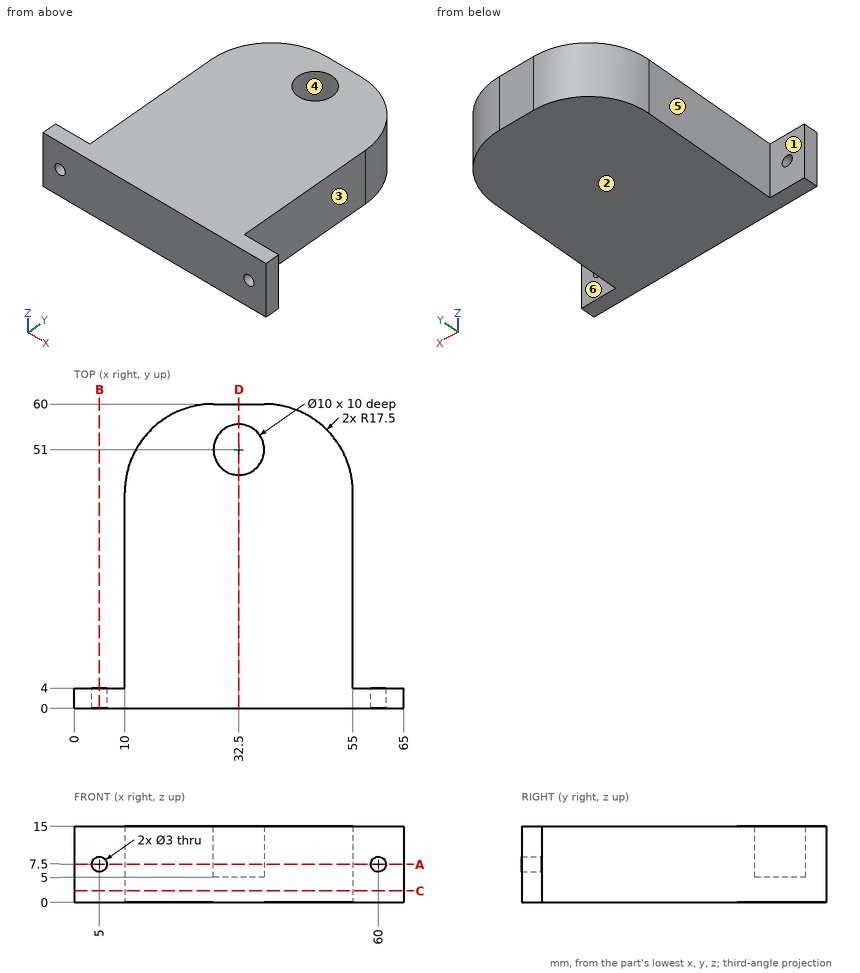
Here's the drawing with two shaded views (mm, measured from the low corner). I have some questions. A direction names the side the tool comes from. Give positions to 0.01 mm unless a question says otherwise; leave off trailing zeros. Order: outer loops, then holes, each group sorted by start corner. A loop starts at its lowest first (then second) coordinate and runs counter-clockwise, first axis right, second up. Notation, with made-up numbers: (5.25, 73.5) -> (39.25, 73.5) arc R23 cw to (39.25, 91.5) -> close; hole circle Ø7 at (19.5, -26). An arc over 180 degrees is marked (long way). One line per item, written item: value. Start each with the question number.
1. For the marked faces 1, 2 and 3, which set-ups out of +Z, -Z, +X, -X, +Y, -Y let a thin tool reach every point of the face, with its end or its side?
2. Imagine slicing it at B-B, the plane x = 5. List the corners of the cut face in (y, z) for me.
3. Imagine slicing it at C-C, the plane z = 2.25. List the corners of the cut face in (x, y) for me, plus the area to 3 significant figures.
4. We'd pull the mould along Y, two halves only. Please class the marked faces 4, 5 and 6: released by +Y, released by -Y, zero draft, split by the parting line, or undercut.
5. I need wall thicknesses on probe 1 along X at (y, z) = (2.65, 7.5); probe 2 along Z at (x, y) = (5, 2.45); probe 3 along X at (y, z) = (28, 9). Which ranges of each line are inside material? Lowest first, please. Write a range as from..to.
6. Will these pins go through, and if not, where does the flat tip stop? pin 1 Ø1 at (x, y) = (17.5, 10) entering from -Z; pin 2 Ø2 at (y, z) = (41, 7.5) entering from -X; pin 3 Ø1 at (y, z) = (47.5, 4) entering from +X; pin 4 Ø5 at (x, z) = (7, 10) entering from +Y.
7. Imagine slicing it at D-D, the plane x = 32.5. List the corners of the cut face in (y, z) for me, plus the area to 3 significant figures.
8. Imagine slicing it at A-A, the plane z = 7.5. List the corners of the cut face in (x, y) for me, plus the area to 3 significant figures.
Values follow:
1. face 1: +Z, -Z, -X, +Y
1. face 2: -Z, +X, -X, +Y, -Y
1. face 3: +Z, -Z, +X, +Y
2. outline: (0, 0) -> (4, 0) -> (4, 6) -> (0, 6) -> close; (0, 9) -> (4, 9) -> (4, 15) -> (0, 15) -> close
3. outline: (0, 0) -> (65, 0) -> (65, 4) -> (55, 4) -> (55, 42.5) arc R17.5 ccw to (37.5, 60) -> (27.5, 60) arc R17.5 ccw to (10, 42.5) -> (10, 4) -> (0, 4) -> close
3. area: 2,650 mm2
4. face 4: undercut
4. face 5: zero draft
4. face 6: released by +Y
5. probe 1: x = 0..3.5, 6.5..58.5, 61.5..65
5. probe 2: z = 0..6, 9..15
5. probe 3: x = 10..55
6. pin 1: stops at z = 0
6. pin 2: stops at x = 10
6. pin 3: stops at x = 54.41
6. pin 4: stops at y = 4
7. outline: (0, 0) -> (60, 0) -> (60, 15) -> (56, 15) -> (56, 5) -> (46, 5) -> (46, 15) -> (0, 15) -> close
7. area: 800 mm2
8. outline: (0, 0) -> (3.5, 0) -> (3.5, 4) -> (0, 4) -> close; (6.5, 0) -> (58.5, 0) -> (58.5, 4) -> (55, 4) -> (55, 42.5) arc R17.5 ccw to (37.5, 60) -> (27.5, 60) arc R17.5 ccw to (10, 42.5) -> (10, 4) -> (6.5, 4) -> close; (61.5, 0) -> (65, 0) -> (65, 4) -> (61.5, 4) -> close; hole circle Ø10 at (32.5, 51)
8. area: 2,550 mm2
